Could you check a few things on this model? Use its own coordinates, in mm. A direction names the side the tool comes from. Round coordinates to 2 decimals unless told otherwise and drop trailing zeros. Loops run counter-clockwise (first coordinate to the right, second up) from the corner with the lowest first, then second, coordinate; pieces in that order, holes last. Notation, with made-up numbers: (33, -38) -> (81, -38) arc R17 cw to (81, -15) -> close; hole circle Ø10 at (69, -19). An arc over 180 degrees is marked (long way). Write each question's results on one line, items separated by ' | '. Start each with the question number.
1) We'd pull the mould along Z, two halves only. Please class faces 3 (the flat face through (0, 4, -21.5)), 4 (the flat face through (-32.5, 4, 0)), 5 (the cylindrical face through (17.292, 2.028, -19.086)), 6 (the cylindrical face through (15.1, 5.9, -15.7)): pulls with the +Z half, pulls with the -Z half, needs draft (parallel to the pull), parting line crosses it, or undercut.
2) Imagine slicing it at B-B, the plane z = -17.5. List the corners of the cut face in (x, y) for me, plus the area to 3 significant figures.
3) Imagine slicing it at C-C, the plane y = 6. List the corners of the cut face in (x, z) for me, plus the area to 3 significant figures.
4) For P1, Ø3.5, axis at x = 17.5, z = 17.5, coming from the +Y side, with a flat end and sliding along its axis, tell me the tip position at first contact or that it passes through.
5) If I drill on probe 1 along X at (y, z) = (1.6, -17.5); probe 2 along Z at (x, y) = (-17.5, 5.95); probe 3 along Z at (x, y) = (-17.5, 2), over which ranges is the centre line in solid material (lowest first)?
6) Which directions (+Z, -Z, +X, -X, +Y, -Y) give clear straight access to the entire face, cutting with the end or side of a thin tool? Please do faces 1 (the flat face through (0, 0, 0)), 2 (the cylindrical face through (-19.9, 5.9, 19.3)).
7) Imagine slicing it at A-A, the plane x = 17.5. List the corners of the cut face in (y, z) for me, plus the area to 3 significant figures.
from build123d import *

# Parameters (mm, degrees)
SKETCH2_W           = 65
SKETCH2_H           = 43
BOSS_EXTRUDE1_DEPTH = 7.8
FILLET1_R           = 1
CUT_EXTRUDE1_REACH  = 9.8
SKETCH3_R           = 1.6
SKETCH4_R           = 3
CUT_EXTRUDE2_DEPTH  = 3.8


with BuildPart() as part:
    # Sketch2 → Boss-Extrude1 (new body)
    with BuildSketch(Plane(origin=(0, 0, 0), x_dir=(1, 0, 0), z_dir=(0, 1, 0))):
        Rectangle(SKETCH2_W, SKETCH2_H)
    extrude(amount=BOSS_EXTRUDE1_DEPTH)

    # Fillet1
    fillet1_edges = [part.edges().sort_by_distance(p)[0] for p in [
        (-32.5, 3.9, -21.5),
        (32.5, 3.9, -21.5),
        (32.5, 3.9, 21.5),
        (-32.5, 3.9, 21.5),
    ]]
    fillet(fillet1_edges, radius=FILLET1_R)

    # Sketch3 → Cut-Extrude1 (cut, up to next)
    with BuildSketch(Plane(origin=(0, 7.8, 0), x_dir=(1, 0, 0), z_dir=(0, 1, 0)), mode=Mode.PRIVATE) as cut_extrude1_sk1:
        with Locations((-17.5, 17.5)):
            Circle(SKETCH3_R)
    cut_extrude1_tool1 = extrude(cut_extrude1_sk1.sketch, amount=-CUT_EXTRUDE1_REACH, mode=Mode.PRIVATE) & part.part
    add(cut_extrude1_tool1.solids().sort_by_distance((-17.5, 7.8, -17.5))[0], mode=Mode.SUBTRACT)
    # Sketch3 → Cut-Extrude1 (cut, up to next)
    with BuildSketch(Plane(origin=(0, 7.8, 0), x_dir=(1, 0, 0), z_dir=(0, 1, 0)), mode=Mode.PRIVATE) as cut_extrude1_sk2:
        with Locations((17.5, 17.5)):
            Circle(SKETCH3_R)
    cut_extrude1_tool2 = extrude(cut_extrude1_sk2.sketch, amount=-CUT_EXTRUDE1_REACH, mode=Mode.PRIVATE) & part.part
    add(cut_extrude1_tool2.solids().sort_by_distance((17.5, 7.8, -17.5))[0], mode=Mode.SUBTRACT)
    # Sketch3 → Cut-Extrude1 (cut, up to next)
    with BuildSketch(Plane(origin=(0, 7.8, 0), x_dir=(1, 0, 0), z_dir=(0, 1, 0)), mode=Mode.PRIVATE) as cut_extrude1_sk3:
        with Locations((17.5, -17.5)):
            Circle(SKETCH3_R)
    cut_extrude1_tool3 = extrude(cut_extrude1_sk3.sketch, amount=-CUT_EXTRUDE1_REACH, mode=Mode.PRIVATE) & part.part
    add(cut_extrude1_tool3.solids().sort_by_distance((17.5, 7.8, 17.5))[0], mode=Mode.SUBTRACT)
    # Sketch3 → Cut-Extrude1 (cut, up to next)
    with BuildSketch(Plane(origin=(0, 7.8, 0), x_dir=(1, 0, 0), z_dir=(0, 1, 0)), mode=Mode.PRIVATE) as cut_extrude1_sk4:
        with Locations((-17.5, -17.5)):
            Circle(SKETCH3_R)
    cut_extrude1_tool4 = extrude(cut_extrude1_sk4.sketch, amount=-CUT_EXTRUDE1_REACH, mode=Mode.PRIVATE) & part.part
    add(cut_extrude1_tool4.solids().sort_by_distance((-17.5, 7.8, 17.5))[0], mode=Mode.SUBTRACT)

    # Sketch4 → Cut-Extrude2 (cut)
    with BuildSketch(Plane(origin=(0, 7.8, 0), x_dir=(1, 0, 0), z_dir=(0, 1, 0))):
        with Locations((-17.5, 17.5)):
            Circle(SKETCH4_R)
        with Locations((17.5, 17.5)):
            Circle(SKETCH4_R)
        with Locations((17.5, -17.5)):
            Circle(SKETCH4_R)
        with Locations((-17.5, -17.5)):
            Circle(SKETCH4_R)
    extrude(amount=-CUT_EXTRUDE2_DEPTH, mode=Mode.SUBTRACT)


solid = part.part
Checked values:
1) face 3: pulls with the -Z half | face 4: needs draft | face 5: undercut | face 6: undercut
2) outline: (-32.5, 0) -> (-19.1, 0) -> (-19.1, 4) -> (-20.5, 4) -> (-20.5, 7.8) -> (-32.5, 7.8) -> close; (-15.9, 0) -> (15.9, 0) -> (15.9, 4) -> (14.5, 4) -> (14.5, 7.8) -> (-14.5, 7.8) -> (-14.5, 4) -> (-15.9, 4) -> close; (19.1, 0) -> (32.5, 0) -> (32.5, 7.8) -> (20.5, 7.8) -> (20.5, 4) -> (19.1, 4) -> close | area: 436 mm^2
3) outline: (-32.5, -20.5) arc R1 ccw to (-31.5, -21.5) -> (31.5, -21.5) arc R1 ccw to (32.5, -20.5) -> (32.5, 20.5) arc R1 ccw to (31.5, 21.5) -> (-31.5, 21.5) arc R1 ccw to (-32.5, 20.5) -> close; hole circle Ø6 at (-17.5, -17.5); hole circle Ø6 at (-17.5, 17.5); hole circle Ø6 at (17.5, -17.5); hole circle Ø6 at (17.5, 17.5) | area: 2,680 mm^2
4) P1: y = 4
5) probe 1: -32.5 to -19.1, -15.9 to 15.9, 19.1 to 32.5 | probe 2: -21.5 to -20.5, -14.5 to 14.5, 20.5 to 21.5 | probe 3: -21.5 to -19.1, -15.9 to 15.9, 19.1 to 21.5
6) face 1: +Z, -Z, +X, -X, -Y | face 2: +Y
7) outline: (0, -21.5) -> (7.8, -21.5) -> (7.8, -20.5) -> (4, -20.5) -> (4, -19.1) -> (0, -19.1) -> close; (0, -15.9) -> (4, -15.9) -> (4, -14.5) -> (7.8, -14.5) -> (7.8, 14.5) -> (4, 14.5) -> (4, 15.9) -> (0, 15.9) -> close; (0, 19.1) -> (4, 19.1) -> (4, 20.5) -> (7.8, 20.5) -> (7.8, 21.5) -> (0, 21.5) -> close | area: 264 mm^2
